from build123d import *

# Parameters (mm, degrees)
F2_W          = 2
F2_H          = 7.5
F3_DEPTH      = 7.496
F3_DEPTH_BACK = 7.496
F4_W          = 2
F4_H          = 7.495
F5_DEPTH      = 8


with BuildPart() as f1:
    # F0 (on Front) → F1 (revolve)
    with BuildSketch(Plane.XZ):
        Polygon((0, 6.25), (0, 4.5), (21, 4.5), (21, 0), (73.3, 0), (73.3, 2.995), (64.3, 2.995), (64.3, 4.475), (46.3, 4.475), (46.3, 4.495), (30, 4.495), (30, 7.28), (22.5, 7.28), (22.5, 7.1), (21.5, 7.1), (21.5, 7.495), (13, 7.495), (13, 7.1), (12, 7.1), (12, 7.495), (10, 7.495), (10, 6.25), align=None)
    revolve(axis=Axis((62.9070794401, 0, 0), (1, 0, 0)))

    # F2 (on Front) → F3 (cut, two sides)
    with BuildSketch(Plane.XZ) as f3_sk:
        with Locations((9, 3.75)):
            Rectangle(F2_W, F2_H)
    extrude(amount=-F3_DEPTH, mode=Mode.SUBTRACT)
    extrude(f3_sk.sketch, amount=F3_DEPTH_BACK, mode=Mode.SUBTRACT)

    # F4 (on face) → F5 (cut, through all)
    with BuildSketch(Plane(origin=(0, 0, 0), x_dir=(0, -1, 0), z_dir=(-1, 0, 0))):
        with Locations((0, 3.7475)):
            Rectangle(F4_W, F4_H)
    extrude(amount=-F5_DEPTH, mode=Mode.SUBTRACT)


solid = f1.part
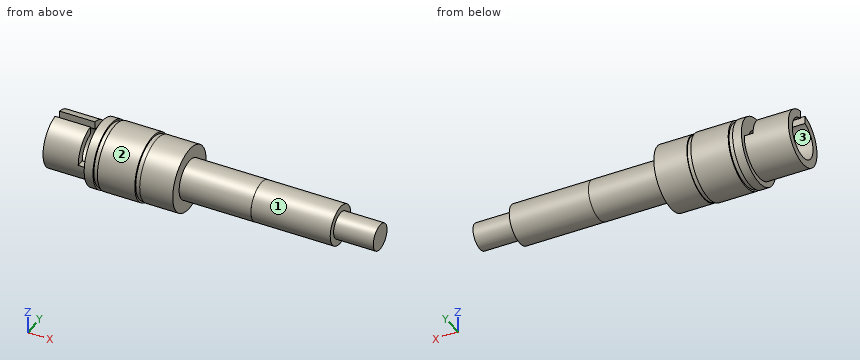
Could you check a few things on this model? Use its own coordinates, in mm. Face numbers are marked on the shaded views. A direction names the side the tool comes from. Give positions to 0.01 mm unless a question says otherwise; leave off trailing zeros. Order: outer loops, then holes, each group sorted by start corner. A loop starts at its lowest first (then second) coordinate and runs counter-clockwise, first axis right, second up. Notation, with made-up numbers: (6, 55.25) - (46, 55.25) arc R15 ccw to (46, 79.25) - close; hole circle Ø11 at (22, -26). An arc over 180 degrees is marked (long way). One line per question, with ' | ' between items. Start each with the question number.
Item 1: For the marked faces 1, 2 and 3, which set-ups out of +Z, -Z, +X, -X, +Y, -Y let a thin tool reach every point of the face, with its end or its side?
Item 2: I'm going to push flat-ended pins straight in: pin 1 Ø6 at (x, z) = (54, 5.5) entering from +Y; pin 2 Ø3 at (y, z) = (-2, -5) entering from +X; pin 3 Ø1.9 at (x, y) = (9.5, -5) entering from +Z. Where does each tip first touch, or does it pass through?
Item 3: I want a section at C-C on z = 1.75. Give the number of separate pieces and of enclosed holes in the cut face, then the cut area to 3 significant figures.
Item 4: I want a section at A-A on x = 18. Write out the boundary of the cut face in (y, z) (3 decimals).
Item 5: I need wall thicknesses on probe 1 along Y at (x, z) = (14, 0) (3 decimals); probe 2 along Y at (x, z) = (7, 0); probe 3 along Z at (x, y) = (6.75, 0). Which ranges of each line are inside material? Lowest first, please. Write a range as [from, to].
Item 6: I want a section at D-D on x = 67.5. Write out the boundary of the cut face in (y, z) (3 decimals), then the cut area to 3 significant figures.
Item 7: I want a section at B-B on x = 31. Write out the boundary of the cut face in (y, z) (3 decimals), then the cut area to 3 significant figures.
Verdict:
1) face 1: +X | face 2: +X, -X | face 3: -X
2) pin 1: y = 3.71 | pin 2: x = 64.3 | pin 3: z = 6.21
3) separate pieces: 3 | enclosed holes: 0 | area: 552 mm^2
4) outline: circle Ø14.99 at (0, 0); hole circle Ø9 at (0, 0)
5) probe 1: [-7.495, -4.5], [4.5, 7.495] | probe 2: [-6.25, -4.5], [4.5, 6.25] | probe 3: [-6.25, -4.5]
6) outline: circle Ø5.99 at (0, 0) | area: 28.2 mm^2
7) outline: circle Ø8.99 at (0, 0) | area: 63.5 mm^2
